Geometry: final body of the model. Coordinates: model frame, mm. A direction names the side the tool comes from. Round coordinates to 2 decimals unless told otherwise and drop trailing zeros. Loops run counter-clockwise (first coordinate to the right, second up) from the corner with the lowest first, then second, coordinate; pieces in that order, holes last. Notation, with made-up numbers: M -24.5,14.5 L 21.5,14.5 A14 ccw 21.5,40.5 Z; hole C 54.5,-29.5 d11. An arc over 180 degrees is marked long. Return JSON: item names as keys, results as strings.
from build123d import *

# Parameters (mm, degrees)
F0_R      = 70
F1_DEPTH  = 191
F3_DEPTH  = 20
F4_R      = 52.5
F5_DEPTH  = 5
F6_R      = 35
F6_R_2    = 32
F7_DEPTH  = 2.5
F9_DEPTH  = 30
F10_W     = 90
F10_H     = 90
F11_DEPTH = 101
F13_W     = 132
F13_H     = 110
F13_R     = 3.75
F14_DEPTH = 8
F15_R     = 5


with BuildPart() as f1:
    # F0 (on Front) → F1 (new body)
    with BuildSketch(Plane.XZ):
        Circle(F0_R)
    extrude(amount=F1_DEPTH)

    # F2 (on face) → F3 (join)
    with BuildSketch(Plane.XZ.offset(191)):
        with BuildLine():
            ThreePointArc((7.5, -59.529404499), (45, -39.686269666), (60, 0))
            ThreePointArc((60, 0), (58.8142780033, 11.8693177122), (55.3039765683, 23.2695117211))
            Line((55.3039765683, 23.2695117211), (47.8039765683, 36.2598927779))
            ThreePointArc((47.8039765683, 36.2598927779), (0, 60), (-47.8039765683, 36.2598927779))
            Line((-47.8039765683, 36.2598927779), (-55.3039765683, 23.2695117211))
            ThreePointArc((-55.3039765683, 23.2695117211), (-51.9615242271, -30), (-7.5, -59.529404499))
            Line((-7.5, -59.529404499), (7.5, -59.529404499))
        make_face()
        with BuildLine():
            Line((47.8039765683, 36.2598927779), (55.3039765683, 23.2695117211))
            ThreePointArc((55.3039765683, 23.2695117211), (51.9615242271, 30), (47.8039765683, 36.2598927779))
        make_face()
        with BuildLine():
            ThreePointArc((47.8039765683, 36.2598927779), (51.9615242271, 30), (55.3039765683, 23.2695117211))
            Line((55.3039765683, 23.2695117211), (63.9642306061, 28.2695117211))
            Line((63.9642306061, 28.2695117211), (56.4642306061, 41.2598927779))
            Line((56.4642306061, 41.2598927779), (47.8039765683, 36.2598927779))
        make_face()
        with BuildLine():
            Line((7.5, -69.529404499), (7.5, -59.529404499))
            ThreePointArc((7.5, -59.529404499), (0, -60), (-7.5, -59.529404499))
            Line((-7.5, -59.529404499), (-7.5, -69.529404499))
            Line((-7.5, -69.529404499), (7.5, -69.529404499))
        make_face()
        with BuildLine():
            ThreePointArc((-7.5, -59.529404499), (0, -60), (7.5, -59.529404499))
            Line((7.5, -59.529404499), (-7.5, -59.529404499))
        make_face()
        with BuildLine():
            Line((-55.3039765683, 23.2695117211), (-47.8039765683, 36.2598927779))
            ThreePointArc((-47.8039765683, 36.2598927779), (-51.9615242271, 30), (-55.3039765683, 23.2695117211))
        make_face()
        with BuildLine():
            ThreePointArc((-55.3039765683, 23.2695117211), (-51.9615242271, 30), (-47.8039765683, 36.2598927779))
            Line((-47.8039765683, 36.2598927779), (-56.4642306061, 41.2598927779))
            Line((-56.4642306061, 41.2598927779), (-63.9642306061, 28.2695117211))
            Line((-63.9642306061, 28.2695117211), (-55.3039765683, 23.2695117211))
        make_face()
    extrude(amount=F3_DEPTH)

    # F4 (on face) → F5 (join)
    with BuildSketch(Plane.XZ.offset(211)):
        Circle(F4_R)
    extrude(amount=F5_DEPTH)

    # F6 (on face) → F7 (join)
    with BuildSketch(Plane.XZ.offset(216)):
        Circle(F6_R)
        Circle(F6_R_2, mode=Mode.SUBTRACT)
    extrude(amount=F7_DEPTH)

    # F8 (on face) → F9 (join)
    with BuildSketch(Plane.XZ.offset(216)):
        with BuildLine():
            ThreePointArc((-2.5, 6.5383484153), (-3.9686269666, -5.7662812973), (7, 0))
            ThreePointArc((7, 0), (5.7662812973, 3.9686269666), (2.5, 6.5383484153))
            Line((2.5, 6.5383484153), (2.5, 4))
            Line((2.5, 4), (-2.5, 4))
            Line((-2.5, 4), (-2.5, 6.5383484153))
        make_face()
        with BuildLine():
            Line((2.5, 4), (2.5, 6.5383484153))
            ThreePointArc((2.5, 6.5383484153), (0, 7), (-2.5, 6.5383484153))
            Line((-2.5, 6.5383484153), (-2.5, 4))
            Line((-2.5, 4), (2.5, 4))
        make_face()
        with BuildLine():
            ThreePointArc((-2.5, 6.5383484153), (0, 7), (2.5, 6.5383484153))
            Line((2.5, 6.5383484153), (2.5, 9))
            Line((2.5, 9), (-2.5, 9))
            Line((-2.5, 9), (-2.5, 6.5383484153))
        make_face()
    extrude(amount=F9_DEPTH)

    # F10 (on Top) → F11 (join)
    with BuildSketch(Plane.XY):
        with Locations((0, -146)):
            Rectangle(F10_W, F10_H)
    extrude(amount=F11_DEPTH)

    # F13 (on offset) → F14 (join)
    with BuildSketch(Plane.XY.offset(-71)):
        with Locations((0, -96)):
            Rectangle(F13_W, F13_H)
        with Locations((-56, -141)):
            Circle(F13_R, mode=Mode.SUBTRACT)
        with Locations((56, -141)):
            Circle(F13_R, mode=Mode.SUBTRACT)
        with Locations((-56, -51)):
            Circle(F13_R, mode=Mode.SUBTRACT)
        with Locations((56, -51)):
            Circle(F13_R, mode=Mode.SUBTRACT)
    extrude(amount=F14_DEPTH)

    # F15
    f15_edges = [f1.edges().sort_by_distance(p)[0] for p in [
        (-70, 0, 0),
        (0, -211, 60),
        (52.134104, -211, 38.759893),
        (59.634104, -211, 25.769512),
        (-51.961524, -211, -30),
        (7.5, -211, -64.529404),
        (0, -211, -69.529404),
        (-7.5, -211, -64.529404),
        (51.961524, -211, -30),
        (-59.634104, -211, 25.769512),
        (-60.214231, -211, 34.764702),
        (-52.134104, -211, 38.759893),
        (-56.464231, -201, 41.259893),
        (-63.964231, -201, 28.269512),
        (56.464231, -201, 41.259893),
        (63.964231, -201, 28.269512),
        (7.5, -201, -69.529404),
        (-7.5, -201, -69.529404),
        (60.214231, -211, 34.764702),
    ]]
    fillet(f15_edges, radius=F15_R)


solid = f1.part
Q1. Section query D-D (y = -175.5). Output: boundary loops of the cut face in (x, z), plus the area to 3 significant figures.
Determined:
{"outline": "M -45,53.62 A70 ccw long 45,53.62 L 45,101 L -45,101 Z", "area": "18,600 mm^2"}
Q2. Reachability of faces 4 (the flat face through (0, -191, 67)), 5 (the cylindrical face through (-52.536, -52.436, -67.056)), 6 (the cylindrical face through (6.07, -209.5, -60.73)) from +Z, -Z, +X, -X, +Y, -Y: full face, straight path, thin tool, end or side. Return the list, or none.
Determined:
{"face 4": "-Y", "face 5": "-Z", "face 6": "-Z, +X, -Y"}
Q3. Material intervals for L1, parallel to Y at x = 56, z = -66; L2, parallel to Z at x = -63, y = -104; L3, parallel to Z at x = 57, y = -99, sorted ascending.
Determined:
{"L1": "y = -151 to -144.75, -137.25 to -54.75, -47.25 to -41", "L2": "z = -71 to -63, -30.51 to 30.51", "L3": "z = -71 to -63, -40.63 to 40.63"}
Q4. Pin query (flat end, axial travel): pin 1 (6 mm diameter, centred on x = 56, y = -51, fed in from +Z); pin 2 (12 mm diameter, centred on x = 56, y = -141, fed in from +Z); pin 3 (6 mm diameter, centred on x = 23.5, y = -34.5, fed in from -Z). Return the tip coordinate at first contact, or that it passes through.
Determined:
{"pin 1": "stops at z = 45.73", "pin 2": "stops at z = 48.99", "pin 3": "stops at z = -66.93"}
Q5. Section query A-A (y = -51). Output: boundary loops of the cut face in (x, z), plus the area to 3 significant figures.
Determined:
{"outline": "M -66,-71 L -59.75,-71 L -59.75,-63 L -66,-63 Z; M -52.25,-71 L 52.25,-71 L 52.25,-63 L 30.51,-63 A70 ccw long -30.51,-63 L -52.25,-63 Z; M 59.75,-71 L 66,-71 L 66,-63 L 59.75,-63 Z", "area": "16,000 mm^2"}
Q6. Section query C-C (z = 80). Output: boundary loops of the cut face in (x, y).
Determined:
{"outline": "M -45,-191 L 45,-191 L 45,-101 L -45,-101 Z"}
Q7. Section query B-B (y = -109). Output: boundary loops of the cut face in (x, z), plus the area to 3 significant figures.
Determined:
{"outline": "M -66,-71 L 66,-71 L 66,-63 L 30.51,-63 A70 ccw 45,53.62 L 45,101 L -45,101 L -45,53.62 A70 ccw -30.51,-63 L -66,-63 Z", "area": "19,400 mm^2"}
Q8. Pull-direction query (Z, two-part tool) for faces 1 (the cylindrical face through (49.56, -209.496, 35.628)), 2 (the flat face through (48, -95, -63)), 3 (the flat face through (11, -216, -34)); classes: pulls with the +Z half, pulls with the -Z half, needs draft (parallel to the pull), parting line crosses it, or undercut.
Determined:
{"face 1": "pulls with the +Z half", "face 2": "undercut", "face 3": "needs draft"}
